Source: three-view drawing plus pictorial views. Frame: mm from the lowest corner of the part. Coordinates: 2 decimals unless noted, no trailing zeros. Order: outer loops, then holes, each group sorted by start corner. A loop starts at its lowest first (then second) coordinate and runs counter-clockwise, first axis right, second up. Notation, with made-up numbers: (37.5, 59) -> (47.5, 59) arc R30 cw to (47.5, 93) -> close; hole circle Ø10 at (20.25, 27.25). An arc over 180 degrees is marked (long way). Use one line per item in the form item = value. Start each with the question number.
1) Pin query (flat end, axial travel): pin 1 (6 mm diameter, centred on y = 160, z = 7.9, fed in from +X); pin 2 (4 mm diameter, centred on y = 110, z = 7.9, fed in from +X); pin 3 (5 mm diameter, centred on x = 170.76, y = 14, fed in from +Z); pin 4 (1.5 mm diameter, centred on y = 160.5, z = 8.5, fed in from -X). Return the tip coordinate at first contact, or that it passes through.
2) Section query C-C on y = 169. Output: boundary loops of the cut face in (x, z), then the cut area to 3 significant figures.
3) Ray query, line 1 along Y through (x, z) = (170.76, 8); line 2 along X through (y, z) = (26.5, 11.25) (1 decimal); line 3 along Z through (x, y) = (8.75, 110). Return the intervals inside material, ascending.
4) Section query A-A on z = 2. Output: boundary loops of the cut face in (x, y) (1 decimal).
5) Section query D-D on x = 306. Output: boundary loops of the cut face in (y, z), then the cut area to 3 significant figures.
6) Section query B-B on x = 252.5. Output: boundary loops of the cut face in (y, z), then the cut area to 3 significant figures.
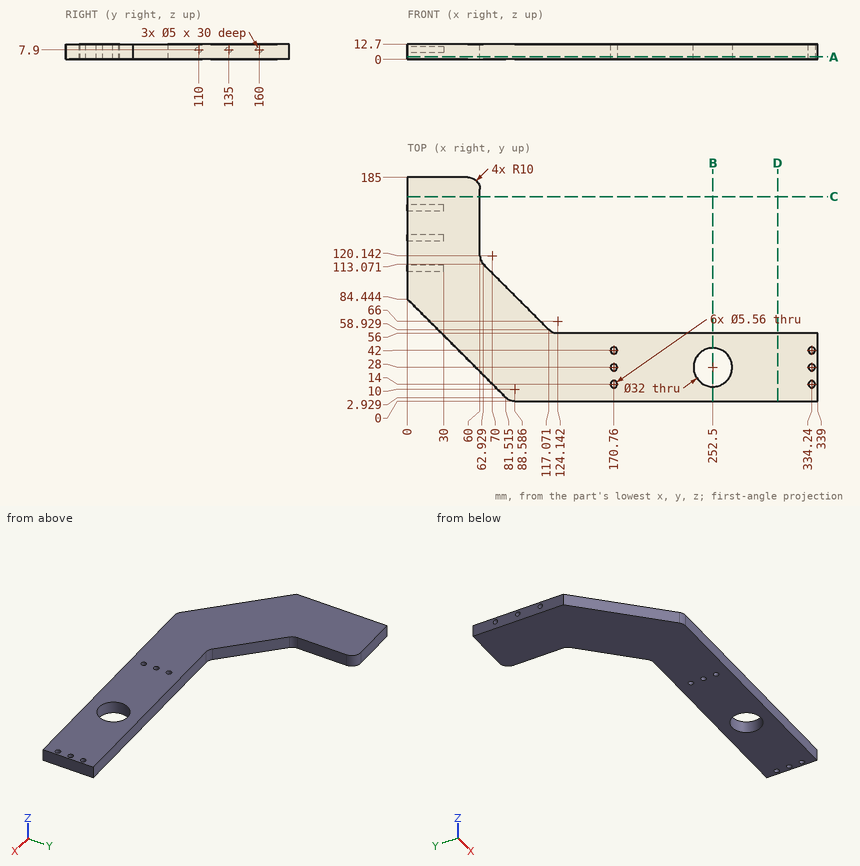
Answers below:
q1.pin_1 = 60
q1.pin_2 = 68
q1.pin_3 = through
q1.pin_4 = 30
q2.outline = (0, 0) -> (60, 0) -> (60, 12.7) -> (0, 12.7) -> close
q2.area = 762 mm^2
q3.line_1 = 0 to 11.22, 16.78 to 25.22, 30.78 to 39.22, 44.78 to 56
q3.line_2 = 57.9 to 168.4, 173.1 to 236.6, 268.4 to 331.9, 336.6 to 339
q3.line_3 = 0 to 5.4, 10.4 to 12.7
q4.outline = (0, 84.4) -> (81.5, 2.9) arc R10 ccw to (88.6, 0) -> (339, 0) -> (339, 56) -> (124.1, 56) arc R10 cw to (117.1, 58.9) -> (62.9, 113.1) arc R10 cw to (60, 120.1) -> (60, 175) arc R10 ccw to (50, 185) -> (0, 185) -> close; hole circle Ø5.6 at (170.8, 14); hole circle Ø5.6 at (170.8, 28); hole circle Ø5.6 at (170.8, 42); hole circle Ø32 at (252.5, 28); hole circle Ø5.6 at (334.2, 14); hole circle Ø5.6 at (334.2, 28); hole circle Ø5.6 at (334.2, 42)
q5.outline = (0, 0) -> (56, 0) -> (56, 12.7) -> (0, 12.7) -> close
q5.area = 711 mm^2
q6.outline = (0, 0) -> (12, 0) -> (12, 12.7) -> (0, 12.7) -> close; (44, 0) -> (56, 0) -> (56, 12.7) -> (44, 12.7) -> close
q6.area = 305 mm^2
